For this review, use the dimensioned drawing (mm, ordinates from the lowest corner) and the shaded views. A direction names the side the tool comes from. Round coordinates to 2 decimals unless told otherwise and drop trailing zeros. Order: outer loops, then holes, each group sorted by start corner. A loop starts at its lowest first (then second) coordinate and runs counter-clockwise, first axis right, second up. Notation, with made-up numbers: M 77,0 L 130,0 A26 cw 130,37 Z; hole C -7.75,46 d3. An arc over 180 degrees is marked long. Use a Markdown table: item, result. Add a question column.
1. Consider section A-A on y = 10. State the section outline as (x, z) points, then the cut area to 3 significant figures.
2. To check wall thickness, follow probe 1 along X at (y, z) = (17.5, 1.75); probe 2 along Y at (x, z) = (22, 10); probe 3 along Z at (x, y) = (28.25, 7). State the ranges of each line that lie inside material, in increasing order.
3. Consider section D-D on y = 17. State the section outline as (x, z) points, then the cut area to 3 significant figures.
4. Consider section C-C on x = 23. State the section outline as (y, z) points, then the cut area to 3 significant figures.
5. For the marked faces 1 and 2, list the 3-axis set-ups (+Z, -Z, +X, -X, +Y, -Y) from which the entire face can be reached by the end or side of a thin tool; tool diameter is ignored.
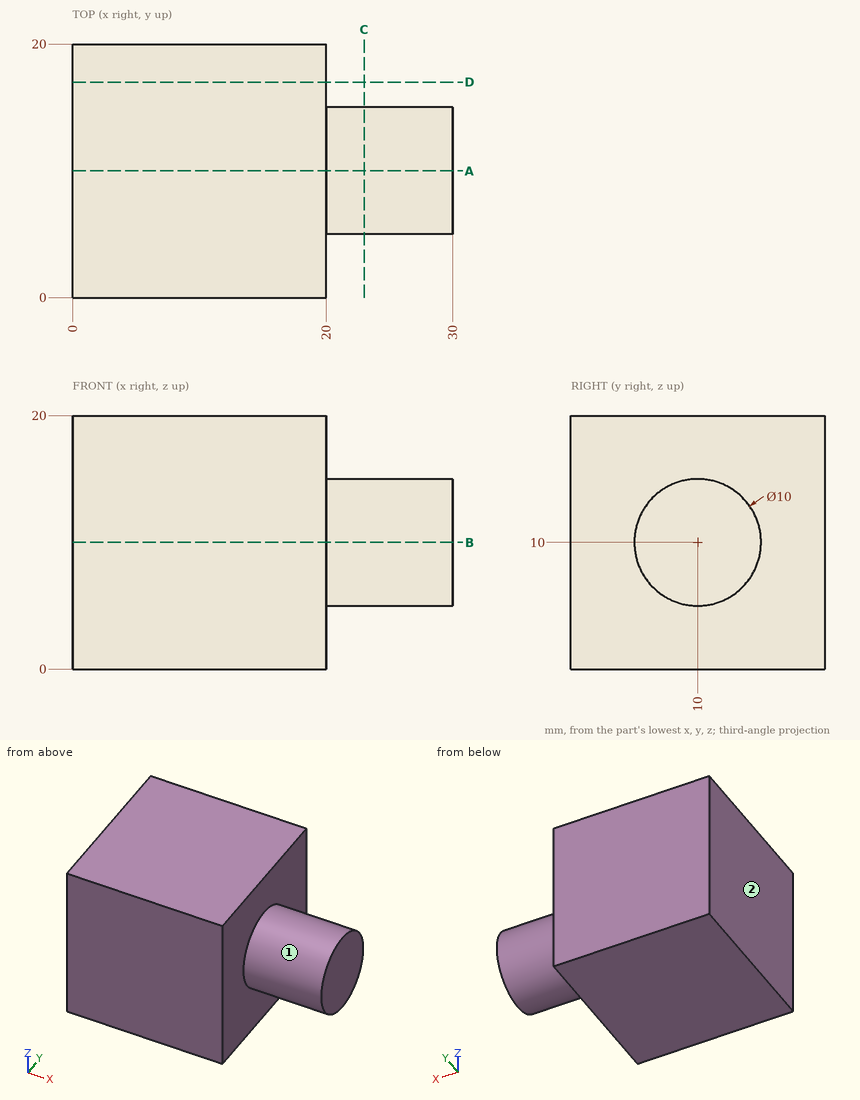
Answer block:
| question | item | result |
|---|---|---|
| 1 | outline | M 0,0 L 20,0 L 20,5 L 30,5 L 30,15 L 20,15 L 20,20 L 0,20 Z |
| 1 | area | 500 mm^2 |
| 2 | probe 1 | 0 to 20 |
| 2 | probe 2 | 5 to 15 |
| 2 | probe 3 | 6 to 14 |
| 3 | outline | M 0,0 L 20,0 L 20,20 L 0,20 Z |
| 3 | area | 400 mm^2 |
| 4 | outline | C 10,10 d10 |
| 4 | area | 78.5 mm^2 |
| 5 | face 1 | +X |
| 5 | face 2 | +Z, -Z, -X, +Y, -Y |
